Design review of the part shown in the three views and the two pictorial views. Dimensions are in mm from the part's minimum x, y and z. Round coordinates to 2 decimals unless told otherwise and drop trailing zeros. Write each loop counter-clockwise with the first axis right and the second up, starting at its lowest first coordinate (ties: lowest second). Pieces come first, ordered by that corner, then holes. Notation, with made-up numbers: (4.25, 23) - (9.25, 23) arc R34 ccw to (9.25, 62) - close; hole circle Ø4 at (49, -17.5). An arc over 180 degrees is marked (long way). One line per item, written item: value. Start each with the question number.
Q1. Clearance check with flat-ended pins moving along their axes: pin 1 Ø3 at (y, z) = (1, 44) entering from -X; pin 2 Ø1.2 at (x, y) = (3.5, 3) entering from -Z. State where each tip first meets the part, or that it passes through.
Q2. For probe 1 along X at (y, z) = (3, 5.5); probe 2 along Z at (x, y) = (26, 5.25); probe 3 along X at (y, z) = (2.5, 15), list the stretches that pass through material, from the lowest coordinate up.
Q3. Add section C-C on x = 22.5. Write out the cut boundary in (y, z), and give its area (3 significant figures).
Q4. Add section D-D on z = 79.1. Write out the cut boundary in (x, y).
Q5. Add section A-A on z = 15. Write out the cut boundary in (x, y).
Q6. Add section B-B on y = 4. Write out the cut boundary in (x, z).
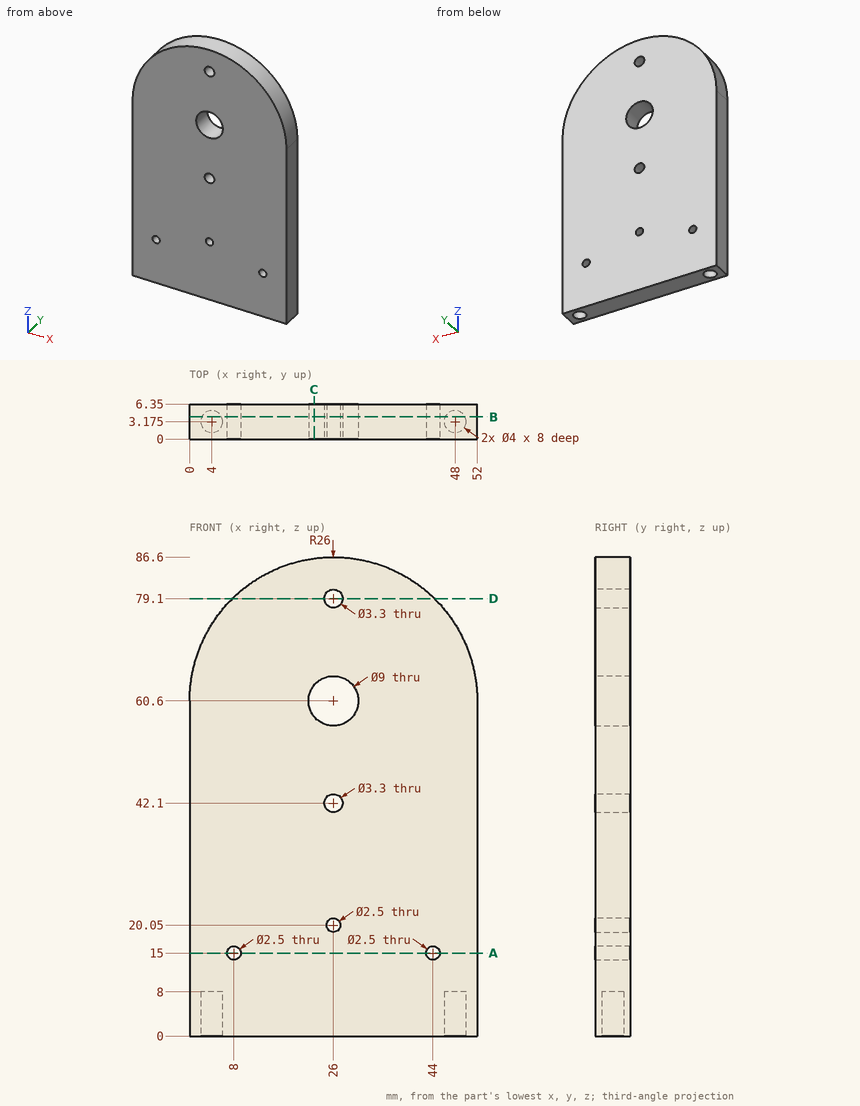
Result set:
1. pin 1: stops at x = 0
1. pin 2: stops at z = 8
2. probe 1: x = 0 to 2.01, 5.99 to 46.01, 49.99 to 52
2. probe 2: z = 0 to 18.8, 21.3 to 40.45, 43.75 to 56.1, 65.1 to 77.45, 80.75 to 86.6
2. probe 3: x = 0 to 6.75, 9.25 to 42.75, 45.25 to 52
3. outline: (0, 0) - (6.35, 0) - (6.35, 57.77) - (0, 57.77) - close; (0, 63.43) - (6.35, 63.43) - (6.35, 86.36) - (0, 86.36) - close
3. area: 512 mm^2
4. outline: (7.73, 0) - (24.35, 0) - (24.35, 6.35) - (7.73, 6.35) - close; (27.65, 0) - (44.27, 0) - (44.27, 6.35) - (27.65, 6.35) - close
5. outline: (0, 0) - (6.75, 0) - (6.75, 6.35) - (0, 6.35) - close; (9.25, 0) - (42.75, 0) - (42.75, 6.35) - (9.25, 6.35) - close; (45.25, 0) - (52, 0) - (52, 6.35) - (45.25, 6.35) - close
6. outline: (0, 0) - (2.18, 0) - (2.18, 8) - (5.82, 8) - (5.82, 0) - (46.18, 0) - (46.18, 8) - (49.82, 8) - (49.82, 0) - (52, 0) - (52, 60.6) arc R26 ccw to (0, 60.6) - close; hole circle Ø2.5 at (8, 15); hole circle Ø9 at (26, 60.6); hole circle Ø3.3 at (26, 42.1); hole circle Ø3.3 at (26, 79.1); hole circle Ø2.5 at (26, 20.05); hole circle Ø2.5 at (44, 15)
